Source: three-view drawing plus pictorial views. Frame: mm from the lowest corner of the part. A direction names the side the tool comes from. Coordinates: 2 decimals unless noted, no trailing zeros. Write each loop counter-clockwise with the first axis right and the second up, starting at its lowest first coordinate (ties: lowest second). Pieces come first, ordered by that corner, then holes. Notation, with made-up numbers: (-14, 66) -> (1, 66) arc R16 cw to (1, 78) -> close; hole circle Ø2 at (17.5, 11). An arc over 180 degrees is marked (long way). One line per question, with ' | ' between items. Start each with the question number.
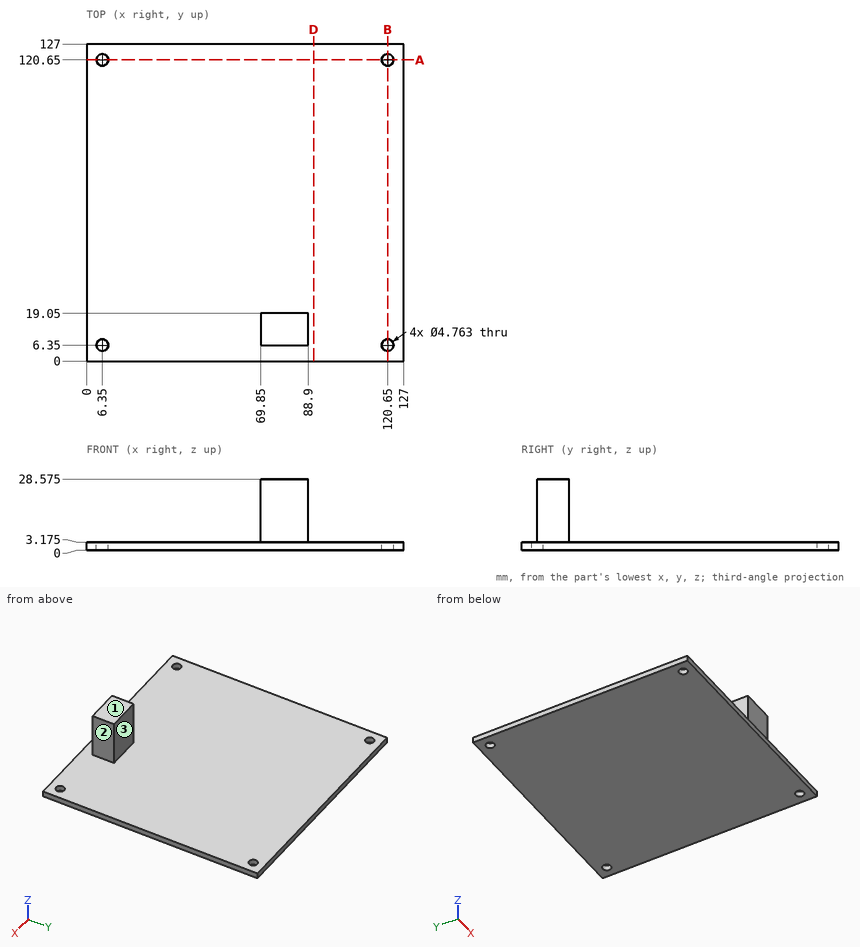
1) Access query for the marked faces 1, 2 and 3. Directions: +Z, -Z, +X, -X, +Y, -Y. A direction counts if a zero-diameter tool reaches every point of the face in a straight line with its end or side. Return the directions, or none.
2) Ray query, line 1 (Y direction, x = 120.65, z = 2.2); line 2 (Z direction, x = 20.5, y = 44) (1 decimal). Return the intervals inside material, ascending.
3) Section A-A, the plane y = 120.65. Return loops of the section in (x, z) (1 decimal).
4) Section D-D, the plane x = 91. Return loops of the section in (y, z) (1 decimal).
5) First-contact query: P1, Ø14, axis at y = 15, z = 13.5, coming from the +X side; P2, Ø8, axis at x = 62.5, y = 24, coming from the +Z side (1 decimal); P3, Ø5, axis at x = 82, z = 12, coming from the -Y side. Flat tips, straight axial feed; report the tip coordinate or a pass-through.
Answer block:
1) face 1: +Z, +X, -X, +Y, -Y | face 2: +Z, +X, +Y, -Y | face 3: +Z, +X, -X, +Y
2) line 1: y = 0 to 3.97, 8.73 to 118.27, 123.03 to 127 | line 2: z = 0 to 3.2
3) outline: (0, 0) -> (4, 0) -> (4, 3.2) -> (0, 3.2) -> close; (8.7, 0) -> (118.3, 0) -> (118.3, 3.2) -> (8.7, 3.2) -> close; (123, 0) -> (127, 0) -> (127, 3.2) -> (123, 3.2) -> close
4) outline: (0, 0) -> (127, 0) -> (127, 3.2) -> (0, 3.2) -> close
5) P1: stops at x = 88.9 | P2: stops at z = 3.2 | P3: stops at y = 6.35
